Geometry check sheet. Reference: the model listing, model coordinates, mm. Face numbers are marked on the shaded views. A direction names the side the tool comes from. Give positions to 0.01 mm unless a question says otherwise; leave off trailing zeros. Write each loop counter-clockwise with the first axis right and the second up, starting at its lowest first coordinate (ties: lowest second). Pieces come first, ordered by that corner, then holes. Notation, with made-up numbers: (72, 37) -> (110, 37) arc R30 cw to (110, 75) -> close; hole circle Ø1 at (60, 24.5). An arc over 180 degrees is marked (long way). One line per item, written item: value.
from build123d import *

# Parameters (mm, degrees)
BOSS_EXTRUDE1_DEPTH                    = 7.5
SKETCH2_4_W                            = 130
SKETCH2_4_H                            = 5
BOSS_EXTRUDE2_DEPTH                    = 50
F_3_0MM_DOWEL_HOLE1_D                  = 3
F_3_0MM_DOWEL_HOLE1_CSINK_D            = 3.05
F_3_0MM_DOWEL_HOLE1_CSINK_ANGLE        = 90
FILLET1_R                              = 5
F_11_5_11_5_DIAMETER_HOLE2_D           = 11.5
F_11_5_11_5_DIAMETER_HOLE2_CSINK_D     = 11.55
F_11_5_11_5_DIAMETER_HOLE2_CSINK_ANGLE = 90
F_1_0_22_DIAMETER_HOLE1_D              = 22
F_1_0_22_DIAMETER_HOLE1_DEPTH          = 140
F_1_0_22_DIAMETER_HOLE1_TIP            = 6.609466809
SKETCH16_W                             = 40
SKETCH16_H                             = 5
BOSS_EXTRUDE3_DEPTH                    = 30
F_3_1_3_1_DIAMETER_HOLE1_AT_2_COUNT    = 2
F_3_1_3_1_DIAMETER_HOLE1_AT_2_PITCH    = 21.505813168
F_3_1_3_1_DIAMETER_HOLE1_AT_3_COUNT    = 2
F_3_1_3_1_DIAMETER_HOLE1_AT_3_PITCH    = 21.505813168
F_3_1_3_1_DIAMETER_HOLE1_AT_4_COUNT    = 2
F_3_1_3_1_DIAMETER_HOLE1_AT_4_PITCH    = 21.505813168
F_3_1_3_1_DIAMETER_HOLE1_AT_5_COUNT    = 2
F_3_1_3_1_DIAMETER_HOLE1_AT_5_PITCH    = 21.505813168
SKETCH22_W                             = 36
SKETCH22_H                             = 24
BOSS_EXTRUDE4_DEPTH                    = 54
SKETCH23_W                             = 28
SKETCH23_H                             = 20
CUT_EXTRUDE1_DEPTH                     = 50
FILLET2_R                              = 4
FILLET3_R                              = 7


with BuildPart() as part:
    # Sketch2 → Boss-Extrude1 (new body)
    with BuildSketch(Plane(origin=(0, 0, 0), x_dir=(1, 0, 0), z_dir=(0, 1, 0))):
        Polygon((65, 65), (-65, 65), (-65, 25.164265249), (-65, 20), (-25, 20), (-25, -20), (-65, -20), (-65, -25.134268309), (-65, -65), (65, -65), align=None)
    extrude(amount=BOSS_EXTRUDE1_DEPTH)

    # Sketch2<4> → Boss-Extrude2 (add)
    with BuildSketch(Plane(origin=(0, 0, 0), x_dir=(1, 0, 0), z_dir=(0, 1, 0))):
        with Locations((0, -67.5)):
            Rectangle(SKETCH2_4_W, SKETCH2_4_H)
        with Locations((0, 67.5)):
            Rectangle(SKETCH2_4_W, SKETCH2_4_H)
    extrude(amount=BOSS_EXTRUDE2_DEPTH)

    # Ø3.0mm Dowel Hole1 (through all)
    with Locations(Plane.XY.offset(70)):
        with Locations((33.2, 28.75), (33.2, 11.25)):
            CounterSinkHole(F_3_0MM_DOWEL_HOLE1_D / 2, F_3_0MM_DOWEL_HOLE1_CSINK_D / 2, counter_sink_angle=F_3_0MM_DOWEL_HOLE1_CSINK_ANGLE)

    # Fillet1
    # the kernel refuses this fillet: 5 mm, written as the material it adds along each edge
    with BuildSketch(Plane(origin=(-65, 7.5, 65), x_dir=(0, 0, -1), z_dir=(1, 0, 0))) as fillet1_piece_1_section:
        with BuildLine():
            CenterArc((FILLET1_R, FILLET1_R), FILLET1_R, 180, 90)
            Line((0, FILLET1_R), (0, 0))
            Line((0, 0), (FILLET1_R, 0))
        make_face()
    fillet1_piece_1 = extrude(amount=130, mode=Mode.PRIVATE)
    fillet1_piece_1 = fillet1_piece_1 - Plane(origin=(33.2, 11.25, 63.865303448), x_dir=(-1, 0, 0), z_dir=(0, 0, -1)) * Cylinder(1.5, 280, mode=Mode.PRIVATE)
    add(fillet1_piece_1)
    with BuildSketch(Plane(origin=(65, 7.5, -65), x_dir=(0, 0, 1), z_dir=(-1, 0, 0))) as fillet1_piece_2_section:
        with BuildLine():
            CenterArc((FILLET1_R, FILLET1_R), FILLET1_R, 180, 90)
            Line((0, FILLET1_R), (0, 0))
            Line((0, 0), (FILLET1_R, 0))
        make_face()
    fillet1_piece_2 = extrude(amount=130, mode=Mode.PRIVATE)
    fillet1_piece_2 = fillet1_piece_2 - Plane(origin=(33.2, 11.25, -63.865303448), x_dir=(-1, 0, 0), z_dir=(0, 0, -1)) * Cylinder(1.5, 280, mode=Mode.PRIVATE)
    add(fillet1_piece_2)

    # Ø11.5 (11.5) Diameter Hole2 (through all)
    with Locations(Plane(origin=(53.8, 20, 70), x_dir=(1, 0, 0), z_dir=(0, 0, 1))):
        with Locations((0, 0)):
            CounterSinkHole(F_11_5_11_5_DIAMETER_HOLE2_D / 2, F_11_5_11_5_DIAMETER_HOLE2_CSINK_D / 2, counter_sink_angle=F_11_5_11_5_DIAMETER_HOLE2_CSINK_ANGLE)

    # Ø1.0 (22) Diameter Hole1
    with Locations(Plane(origin=(-26.2, 20, 70), x_dir=(1, 0, 0), z_dir=(0, 0, 1))):
        with Locations((0, 0)):
            Hole(F_1_0_22_DIAMETER_HOLE1_D / 2, depth=F_1_0_22_DIAMETER_HOLE1_DEPTH)
            with Locations((0, 0, -(F_1_0_22_DIAMETER_HOLE1_DEPTH + F_1_0_22_DIAMETER_HOLE1_TIP / 2))):  # 118° drill point
                Cone(0, F_1_0_22_DIAMETER_HOLE1_D / 2, F_1_0_22_DIAMETER_HOLE1_TIP, mode=Mode.SUBTRACT)

    # Sketch16 → Boss-Extrude3 (add)
    with BuildSketch(Plane(origin=(0, 7.5, 0), x_dir=(1, 0, 0), z_dir=(0, 1, 0))):
        Polygon((-65, 20), (-65, 25.164265249), (-25, 25), (-25, 20), align=None)
        with Locations((-45, -22.5)):
            Rectangle(SKETCH16_W, SKETCH16_H)
    extrude(amount=BOSS_EXTRUDE3_DEPTH)

    # Sketch20 → Ø3.1 (3.1) Diameter Hole1 (revolve, cut)
    with BuildSketch(Plane(origin=(-45, 22.5, -25.082132625), x_dir=(-0.9999915678966332, 0, -0.004106596599781751), z_dir=(0, 1, 0))):
        Polygon((0, 0), (0, 51.096180316), (1.55, 50.164846357), (1.55, 0.025), (1.575, 0), align=None)
    f_3_1_3_1_diameter_hole1 = revolve(axis=Axis((-44.973923112, 22.5, -31.432079081), (-0.004106596599781799, 0, 0.9999915678966332)), mode=Mode.SUBTRACT)

    # Ø3.1 (3.1) Diameter Hole1 at 2: Ø3.1 (3.1) Diameter Hole1 ×2
    with Locations(*[Vector(0.8137266097219926, 0.5812381937190964, 0.0033416751059861844) * (i * F_3_1_3_1_DIAMETER_HOLE1_AT_2_PITCH) for i in range(1, F_3_1_3_1_DIAMETER_HOLE1_AT_2_COUNT)]):
        add(f_3_1_3_1_diameter_hole1, mode=Mode.SUBTRACT)

    # Ø3.1 (3.1) Diameter Hole1 at 3: Ø3.1 (3.1) Diameter Hole1 ×2
    with Locations(*[Vector(-0.8137266097219932, 0.5812381937190956, -0.0033416751059863045) * (i * F_3_1_3_1_DIAMETER_HOLE1_AT_3_PITCH) for i in range(1, F_3_1_3_1_DIAMETER_HOLE1_AT_3_COUNT)]):
        add(f_3_1_3_1_diameter_hole1, mode=Mode.SUBTRACT)

    # Ø3.1 (3.1) Diameter Hole1 at 4: Ø3.1 (3.1) Diameter Hole1 ×2
    with Locations(*[Vector(-0.8137266097219928, -0.5812381937190962, -0.0033416751059863027) * (i * F_3_1_3_1_DIAMETER_HOLE1_AT_4_PITCH) for i in range(1, F_3_1_3_1_DIAMETER_HOLE1_AT_4_COUNT)]):
        add(f_3_1_3_1_diameter_hole1, mode=Mode.SUBTRACT)

    # Ø3.1 (3.1) Diameter Hole1 at 5: Ø3.1 (3.1) Diameter Hole1 ×2
    with Locations(*[Vector(0.8137266097219922, -0.581238193719097, 0.003341675105986184) * (i * F_3_1_3_1_DIAMETER_HOLE1_AT_5_PITCH) for i in range(1, F_3_1_3_1_DIAMETER_HOLE1_AT_5_COUNT)]):
        add(f_3_1_3_1_diameter_hole1, mode=Mode.SUBTRACT)

    # Sketch22 → Boss-Extrude4 (add)
    with BuildSketch(Plane.ZY.offset(65)):
        with Locations((-45.082132625, 19.5)):
            Rectangle(SKETCH22_W, SKETCH22_H)
    extrude(amount=-BOSS_EXTRUDE4_DEPTH)

    # Sketch23 → Cut-Extrude1 (cut)
    with BuildSketch(Plane(origin=(-11, 0, 0), x_dir=(0, 0, -1), z_dir=(1, 0, 0))):
        with Locations((45.082132625, 17.5)):
            Rectangle(SKETCH23_W, SKETCH23_H)
    extrude(amount=-CUT_EXTRUDE1_DEPTH, mode=Mode.SUBTRACT)

    # Fillet2
    fillet2_edges = [part.edges().sort_by_distance(p)[0] for p in [
        (-36, 27.5, -31.082132625),
        (-36, 27.5, -59.082132625),
    ]]
    fillet(fillet2_edges, radius=FILLET2_R)

    # Fillet3
    fillet3_edges = [part.edges().sort_by_distance(p)[0] for p in [
        (-38, 31.5, -27.082132625),
        (-38, 31.5, -63.082132625),
    ]]
    fillet(fillet3_edges, radius=FILLET3_R)


solid = part.part
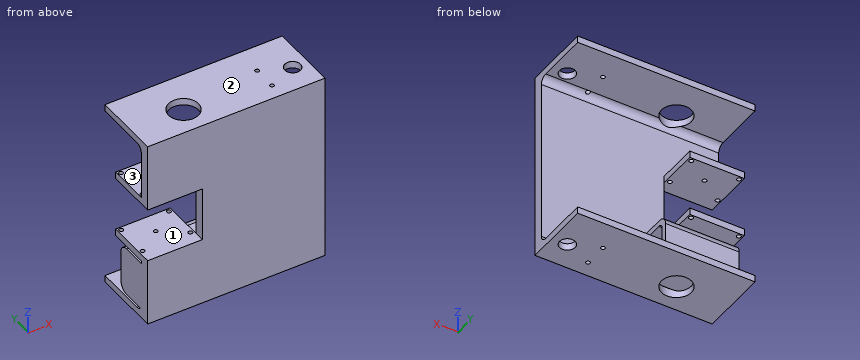
1) Scan lines: probe 1 along Y at (x, z) = (33, -67); probe 2 along X at (y, z) = (20, 67.3); probe 3 along Z at (x, y) = (-34, 16). Record each from-to range of solid material in increasing order.
Verdict:
probe 1: 0 to 9.76, 12.74 to 27.26, 30.24 to 50
probe 2: -65 to -37.2, -15.2 to 48.05, 59.55 to 65
probe 3: -63.08 to -59.08, -31.08 to -27.08, -25.04 to -20, 20 to 25
2) Sectioned sample at B-B on y = 45. Record the cut outline in (x, z).
Verdict:
outline: (-65, -70) -> (65, -70) -> (65, -65) -> (-65, -65) -> close; (-65, 65) -> (65, 65) -> (65, 70) -> (-65, 70) -> close
3) Tool access check on the marked faces 1, 2 and 3. Record the directions out of +Z, -Z, +X, -X, +Y, -Y that give a thin tool (end or side, any length) a straight path to the whole face; none if there is none.
Verdict:
face 1: -X, +Y, -Y
face 2: +Z, +X, -X, +Y, -Y
face 3: +X, -X, +Y
4) Sectioned sample at A-A on x = 53.8. Record the cut outline in (y, z) (3 decimals).
Verdict:
outline: (0, -70) -> (14.25, -70) -> (14.25, -65) -> (12.5, -65) arc R5 cw to (7.5, -60) -> (7.5, 60) arc R5 cw to (12.5, 65) -> (14.25, 65) -> (14.25, 69.975) -> (14.225, 70) -> (0, 70) -> close; (25.75, -70) -> (50, -70) -> (50, -65) -> (25.75, -65) -> close; (25.75, 65) -> (50, 65) -> (50, 70) -> (25.775, 70) -> (25.75, 69.975) -> close
5) Sectioned sample at D-D on x = -48.5. Give the number of separate pieces and of enclosed holes in the cut face, plus the area to 3 significant figures.
Verdict:
separate pieces: 2
enclosed holes: 1
area: 1,780 mm^2
6) Depth check by flat-ended pin: pin 1 Ø13 at (x, y) = (-26.2, 20) entering from -Z; pin 2 Ø6.5 at (x, z) = (-46, -39.5) entering from +Y; pin 3 Ø2.5 at (y, z) = (26.5, 22.5) entering from +X. Enter the tip coordinate at first touch or a pass-through.
Verdict:
pin 1: z = -63.08
pin 2: y = 31.5
pin 3: x = -25
7) Sectioned sample at C-C on x = 12. Record the cut outline in (y, z), plus the area to 3 significant figures.
Verdict:
outline: (0, -70) -> (50, -70) -> (50, -65) -> (12.5, -65) arc R5 cw to (7.5, -60) -> (7.5, 60) arc R5 cw to (12.5, 65) -> (50, 65) -> (50, 70) -> (0, 70) -> close
area: 1,490 mm^2
